from build123d import *

# Parameters (mm, degrees)
SKETCH1_W           = 31.8
SKETCH1_H           = 15.8
BOSS_EXTRUDE1_DEPTH = 9.6
SKETCH2_R           = 2.4
BOSS_EXTRUDE2_DEPTH = 1.8
CUT_EXTRUDE3_DEPTH  = 8.6
SKETCH7_R           = 1.3
CUT_EXTRUDE4_DEPTH  = 1.7
SKETCH8_R           = 3.25
SKETCH8_R_2         = 2.05
BOSS_EXTRUDE4_DEPTH = 8.6
BOSS_EXTRUDE5_DEPTH = 6.3


with BuildPart() as part:
    # Sketch1 → Boss-Extrude1 (new body)
    with BuildSketch(Plane.XY):
        Rectangle(SKETCH1_W, SKETCH1_H)
    extrude(amount=BOSS_EXTRUDE1_DEPTH)

    # Sketch2 → Boss-Extrude2 (add)
    with BuildSketch(Plane.XY.offset(9.6)):
        with Locations((-12, 4)):
            Circle(SKETCH2_R)
        with Locations((-4, 4)):
            Circle(SKETCH2_R)
        with Locations((4, 4)):
            Circle(SKETCH2_R)
        with Locations((12, 4)):
            Circle(SKETCH2_R)
        with Locations((-4, -4)):
            Circle(SKETCH2_R)
        with Locations((4, -4)):
            Circle(SKETCH2_R)
        with Locations((12, -4)):
            Circle(SKETCH2_R)
        with Locations((-12, -4)):
            Circle(SKETCH2_R)
    extrude(amount=BOSS_EXTRUDE2_DEPTH)

    # Sketch6 → Cut-Extrude3 (cut)
    with BuildSketch(Plane(origin=(0, 0, 0), x_dir=(-1, 0, 0), z_dir=(0, 0, -1))):
        Polygon((-14.7, -4.6), (-14.7, -6.7), (-12.6, -6.7), (-12.6, -6.5), (-11.4, -6.5), (-11.4, -6.7), (-4.6, -6.7), (-4.6, -6.5), (-3.4, -6.5), (-3.4, -6.7), (3.4, -6.7), (3.4, -6.5), (4.6, -6.5), (4.6, -6.7), (11.4, -6.7), (11.4, -6.5), (12.6, -6.5), (12.6, -6.7), (14.7, -6.7), (14.7, -4.6), (14.5, -4.6), (14.5, -3.4), (14.7, -3.4), (14.7, 3.4), (14.5, 3.4), (14.5, 4.6), (14.7, 4.6), (14.7, 6.7), (12.6, 6.7), (12.6, 6.5), (11.4, 6.5), (11.4, 6.7), (4.6, 6.7), (4.6, 6.5), (3.4, 6.5), (3.4, 6.7), (-3.4, 6.7), (-3.4, 6.5), (-4.6, 6.5), (-4.6, 6.7), (-11.4, 6.7), (-11.4, 6.5), (-12.6, 6.5), (-12.6, 6.7), (-14.7, 6.7), (-14.7, 4.6), (-14.5, 4.6), (-14.5, 3.4), (-14.7, 3.4), (-14.7, -3.4), (-14.5, -3.4), (-14.5, -4.6), align=None)
    extrude(amount=-CUT_EXTRUDE3_DEPTH, mode=Mode.SUBTRACT)

    # Sketch7 → Cut-Extrude4 (cut)
    with BuildSketch(Plane(origin=(0, 0, 8.6), x_dir=(-1, 0, 0), z_dir=(0, 0, -1))):
        with Locations((-12, 4)):
            Circle(SKETCH7_R)
        with Locations((-4, 4)):
            Circle(SKETCH7_R)
        with Locations((4, 4)):
            Circle(SKETCH7_R)
        with Locations((12, 4)):
            Circle(SKETCH7_R)
        with Locations((-4, -4)):
            Circle(SKETCH7_R)
        with Locations((4, -4)):
            Circle(SKETCH7_R)
        with Locations((12, -4)):
            Circle(SKETCH7_R)
        with Locations((-12, -4)):
            Circle(SKETCH7_R)
    extrude(amount=-CUT_EXTRUDE4_DEPTH, mode=Mode.SUBTRACT)

    # Sketch8 → Boss-Extrude4 (add)
    with BuildSketch(Plane(origin=(0, 0, 8.6), x_dir=(-1, 0, 0), z_dir=(0, 0, -1))):
        with Locations((-8, 0)):
            Circle(SKETCH8_R)
        with Locations((-8, 0)):
            Circle(SKETCH8_R_2, mode=Mode.SUBTRACT)
        Circle(SKETCH8_R)
        Circle(SKETCH8_R_2, mode=Mode.SUBTRACT)
        with Locations((8, 0)):
            Circle(SKETCH8_R)
        with Locations((8, 0)):
            Circle(SKETCH8_R_2, mode=Mode.SUBTRACT)
    extrude(amount=BOSS_EXTRUDE4_DEPTH)

    # Sketch9 → Boss-Extrude5 (add)
    with BuildSketch(Plane(origin=(0, 0, 8.6), x_dir=(-1, 0, 0), z_dir=(0, 0, -1))):
        with BuildLine():
            ThreePointArc((0.55, 3.203123476), (0, 3.25), (-0.55, 3.203123476))
            Line((-0.55, 3.203123476), (-0.55, 6.7))
            Line((-0.55, 6.7), (0.55, 6.7))
            Line((0.55, 6.7), (0.55, 3.203123476))
        make_face()
        with BuildLine():
            ThreePointArc((-0.55, -3.203123476), (0, -3.25), (0.55, -3.203123476))
            Line((0.55, -3.203123476), (0.55, -6.7))
            Line((0.55, -6.7), (-0.55, -6.7))
            Line((-0.55, -6.7), (-0.55, -3.203123476))
        make_face()
    extrude(amount=BOSS_EXTRUDE5_DEPTH)


solid = part.part
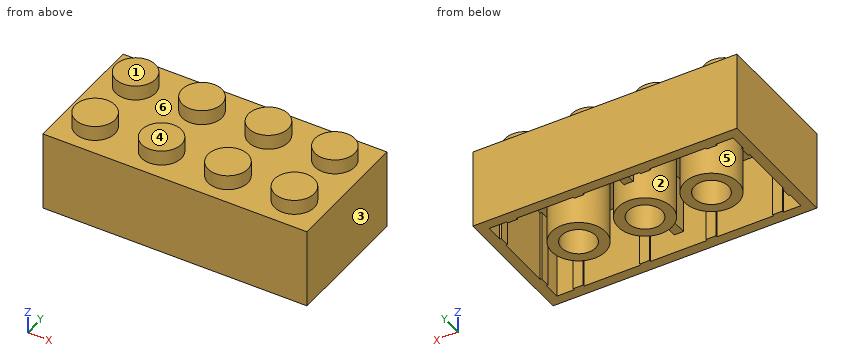
Build history of the part. All positions in model axes, mm. Face numbers are marked on the shaded views. A direction names the side the tool comes from. Round coordinates to 2 decimals unless told otherwise and drop trailing zeros. Loops run counter-clockwise (first coordinate to the right, second up) from the corner with the lowest first, then second, coordinate; pieces in that order, holes last. Notation, with made-up numbers: (-26, 51.5) -> (-4, 51.5) arc R18 cw to (-4, 57.5) -> close; hole circle Ø7 at (87, -1). An arc over 180 degrees is marked (long way). Use CSV: the item, a comma, the result in double quotes. Start each with the question number.
Q1. Mould opens along X. For the marked faces 1, 2 and 3 say: +X half, -X half, draft (parallel to the pull), parting line (faces both ways), or undercut.
Q2. Which spindle directions (+Z, -Z, +X, -X, +Y, -Y) get a long thin tool onto all of the face, cutting with end or side? Do the marked faces 4, 5 and 6. Say none if no direction does.
Q3. Drill centre lines: L1, parallel to X at y = -4.75, z = 4; L2, parallel to Y at x = 0, z = 2; L3, parallel to Y at x = 12, z = 9.9. Where is each one in solid material? Low to high.
Q4. Saw through at A-A on z = 7. Count the separate pieces of the cut face and the enclosed holes in it, and give its area (3 significant figures).
Q5. Saw through at D-D on x = -12. Give the cut face in (y, z), and give its area (3 significant figures).
Q6. Flat gauge pins, fed straight in: pin 1 Ø2 at (x, y) = (-4, -4) entering from -Z; pin 2 Ø3 at (x, y) = (-12.5, -3.5) entering from -Z. Where does each tip first touch, or does it go through?
Q7. Saw through at B-B on x = 8. Give the cut face in (y, z).
Solutions:
1,face 1,"draft"
1,face 2,"undercut"
1,face 3,"+X half"
2,face 4,"+Z, +X, -X, +Y, -Y"
2,face 5,"-Z"
2,face 6,"+Z"
3,L1,"x = -15.9 to -14.7, -0.55 to 0.55, 14.7 to 15.9"
3,L2,"y = -7.9 to -6.7, -3.25 to -2.05, 2.05 to 3.25, 6.7 to 7.9"
3,L3,"y = -6.4 to -5.3, -2.7 to -1.6, 1.6 to 2.7, 5.3 to 6.4"
4,separate pieces,"3"
4,enclosed holes,"5"
4,area,"179 mm^2"
5,outline,"(-7.9, 0) -> (-6.5, 0) -> (-6.5, 8.6) -> (-5.3, 8.6) -> (-5.3, 10.3) -> (-2.7, 10.3) -> (-2.7, 8.6) -> (2.7, 8.6) -> (2.7, 10.3) -> (5.3, 10.3) -> (5.3, 8.6) -> (6.5, 8.6) -> (6.5, 0) -> (7.9, 0) -> (7.9, 9.6) -> (6.4, 9.6) -> (6.4, 11.4) -> (1.6, 11.4) -> (1.6, 9.6) -> (-1.6, 9.6) -> (-1.6, 11.4) -> (-6.4, 11.4) -> (-6.4, 9.6) -> (-7.9, 9.6) -> close"
5,area,"48.3 mm^2"
6,pin 1,"stops at z = 10.3"
6,pin 2,"stops at z = 8.6"
7,outline,"(-7.9, 0) -> (-6.7, 0) -> (-6.7, 8.6) -> (-3.25, 8.6) -> (-3.25, 0) -> (-2.05, 0) -> (-2.05, 8.6) -> (2.05, 8.6) -> (2.05, 0) -> (3.25, 0) -> (3.25, 8.6) -> (6.7, 8.6) -> (6.7, 0) -> (7.9, 0) -> (7.9, 9.6) -> (-7.9, 9.6) -> close"
